Study the drawing (mm; zero at the part's minimum x, y, z) and answer. A direction names the side the tool comes from. Give positions to 0.01 mm unless a question says otherwise; leave off trailing zeros. Loops run counter-clockwise (first coordinate to the right, second up) from the corner with the lowest first, then second, coordinate; pieces in that order, holes last. Notation, with made-up numbers: (51.5, -23) - (106.5, -23) arc R25 cw to (106.5, 5) - close; hole circle Ø2 at (-27.5, 17). An arc over 180 degrees is marked (long way). Answer in a Markdown table with one row per item. Add a question column.
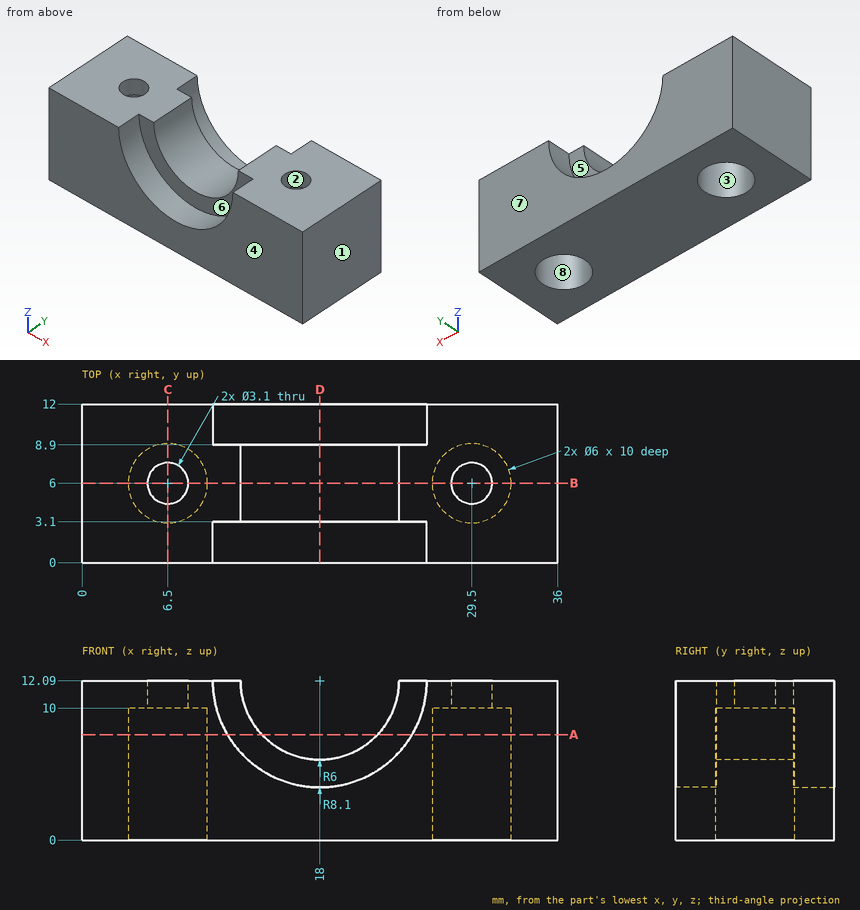
(1) A cutting plane is placed at A-A on z = 8. Determine the outline of the cut face in (x, y).
(2) Find the intervals of material crossed by line 1 along Y through (x, z) = (6.5, 3.5); line 2 along Y through (x, z) = (29.5, 10.9); line 3 along X through (y, z) = (8.25, 0.5), in increasing order. Write a range as [from, to].
(3) A cutting plane is placed at D-D on x = 18. Determine the outline of the cut face in (y, z), plus the area to 3 significant figures.
(4) The mould has two halves that part along Y. Classify the marked faces 1, 2, 3 and 4: pulls with the +Y half, pulls with the -Y half, needs draft (parallel to the pull), parting line crosses it, or undercut.
(5) Given pin 1 Ø3.5 at (x, y) = (6.5, 6) entering from -Z; pin 2 Ø5 at (x, y) = (29.5, 6) entering from +Z, each flat-ended and moving along its own axis, determine where each tip first touches the part or whether it passes through.
(6) A cutting plane is placed at C-C on x = 6.5. Determine the outline of the cut face in (y, z), plus the area to 3 significant figures.
(7) A tool of negligible diameter and unlimited length cuts with its end or side. For the marked faces 5, 6, 7 and 8, from which of +Z, -Z, +X, -X, +Y, -Y can it reach the whole face along a straight path? Write none if from no direction.
(8) A cutting plane is placed at B-B on y = 6. Determine the outline of the cut face in (x, z), plus the area to 3 significant figures.
Evaluation:
| question | item | result |
|---|---|---|
| 1 | outline | (0, 0) - (11.01, 0) - (11.01, 3.1) - (13.61, 3.1) - (13.61, 8.9) - (11.01, 8.9) - (11.01, 12) - (0, 12) - close; (22.39, 3.1) - (24.99, 3.1) - (24.99, 0) - (36, 0) - (36, 12) - (24.99, 12) - (24.99, 8.9) - (22.39, 8.9) - close; hole circle Ø6 at (6.5, 6); hole circle Ø6 at (29.5, 6) |
| 2 | line 1 | y = [0, 3], [9, 12] |
| 2 | line 2 | y = [0, 4.45], [7.55, 12] |
| 2 | line 3 | x = [0, 4.52], [8.48, 27.52], [31.48, 36] |
| 3 | outline | (0, 0) - (12, 0) - (12, 3.99) - (8.9, 3.99) - (8.9, 6.09) - (3.1, 6.09) - (3.1, 3.99) - (0, 3.99) - close |
| 3 | area | 60.1 mm² |
| 4 | face 1 | needs draft |
| 4 | face 2 | undercut |
| 4 | face 3 | undercut |
| 4 | face 4 | pulls with the -Y half |
| 5 | pin 1 | stops at z = 10 |
| 5 | pin 2 | stops at z = 12.09 |
| 6 | outline | (0, 0) - (3, 0) - (3, 10) - (4.45, 10) - (4.45, 12.09) - (0, 12.09) - close; (7.55, 10) - (9, 10) - (9, 0) - (12, 0) - (12, 12.09) - (7.55, 12.09) - close |
| 6 | area | 78.6 mm² |
| 7 | face 5 | +Z, +Y |
| 7 | face 6 | +Z, -Y |
| 7 | face 7 | +Z, -Z, +X, -X, +Y |
| 7 | face 8 | -Z |
| 8 | outline | (0, 0) - (3.5, 0) - (3.5, 10) - (4.95, 10) - (4.95, 12.09) - (0, 12.09) - close; (8.05, 10) - (9.5, 10) - (9.5, 0) - (26.5, 0) - (26.5, 10) - (27.95, 10) - (27.95, 12.09) - (24, 12.09) arc R6 cw to (12, 12.09) - (8.05, 12.09) - close; (31.05, 10) - (32.5, 10) - (32.5, 0) - (36, 0) - (36, 12.09) - (31.05, 12.09) - close |
| 8 | area | 246 mm² |
